Build history of the part. All positions in model axes, mm. Face numbers are marked on the shaded views. A direction names the side the tool comes from. Coordinates: 2 decimals unless noted, no trailing zeros. Loops run counter-clockwise (first coordinate to the right, second up) from the corner with the lowest first, then second, coordinate; pieces in that order, holes last.
Item 1: Cut at A-A (x = 4.5). List the corners of the cut face in (y, z).
Item 2: Cut at B-B (z = 4). List the corners of the cut face in (x, y).
Item 3: 3-axis set-ups, long thin cutter, end or side, ignore diameter. For the marked faces 1, 2 and 3: which of +Z, -Z, +X, -X, +Y, -Y reach the whole face in a straight line?
Item 4: Cut at D-D (x = 0.5). List the corners of the cut face in (y, z).
Item 5: Flat gauge pins, fed straight in: pin 1 (0.6 mm diameter, centred on x = 0.5, y = 17.5, fed in from -Z); pin 2 (1.6 mm diameter, centred on y = 16, z = 16.5, fed in from +X); pin 3 (1.6 mm diameter, centred on x = 4.5, z = 4, fed in from -Y); pin 4 (3.5 mm diameter, centred on y = 15.7, z = 26, fed in from -X). Where does each tip first touch, or does it go through?
Item 6: Mould opens along Y. For the marked faces 4, 5 and 6 say: released by +Y, released by -Y, zero draft, split by the parting line, or undercut.
Item 7: Cut at C-C (z = 20). List the corners of the cut face in (x, y), and give its area (3 significant figures).
Item 8: Drill centre lines: line 1 along Z through (x, y) = (3.6, 15.7); line 2 along Y through (x, z) = (3.25, 25.75); line 3 along Z through (x, y) = (2.75, 16.75). Where is each one in solid material? Low to high.
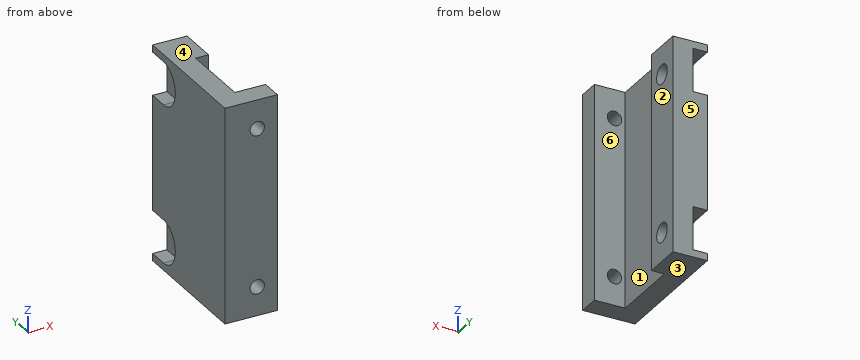
from build123d import *

# Parameters (mm, degrees)
EXTRUDE_1_DEPTH     = 30
CUT_EXTRUDE_1_REACH = 37.994
SKETCH_2_R          = 1
CUT_EXTRUDE_2_REACH = 37.994
SKETCH_3_R          = 1.35
CUT_EXTRUDE_3_DEPTH = 2


with BuildPart() as part:
    # 草图1 → 凸台-拉伸1 (new body)
    with BuildSketch(Plane.XY):
        Polygon((0, 0), (7.3, 0), (7.3, 3), (3, 3), (3, 13), (4.8, 13), (4.8, 18.5), (0, 18.5), align=None)
    extrude(amount=EXTRUDE_1_DEPTH)

    # 草图2 → 切除-拉伸1 (cut, up to next)
    with BuildSketch(Plane.XZ, mode=Mode.PRIVATE) as cut_extrude_1_sk1:
        with Locations((4.5, 26)):
            Circle(SKETCH_2_R)
    cut_extrude_1_tool1 = extrude(cut_extrude_1_sk1.sketch, amount=-CUT_EXTRUDE_1_REACH, mode=Mode.PRIVATE) & part.part
    # 草图2 → 切除-拉伸1 (cut, up to next)
    with BuildSketch(Plane.XZ, mode=Mode.PRIVATE) as cut_extrude_1_sk2:
        with Locations((4.5, 4)):
            Circle(SKETCH_2_R)
    cut_extrude_1_tool2 = extrude(cut_extrude_1_sk2.sketch, amount=-CUT_EXTRUDE_1_REACH, mode=Mode.PRIVATE) & part.part
    add(cut_extrude_1_tool1.solids().sort_by_distance((4.5, 0, 26))[0], mode=Mode.SUBTRACT)
    add(cut_extrude_1_tool2.solids().sort_by_distance((4.5, 0, 4))[0], mode=Mode.SUBTRACT)

    # 草图3 → 切除-拉伸2 (cut, up to next)
    with BuildSketch(Plane.ZY, mode=Mode.PRIVATE) as cut_extrude_2_sk1:
        with Locations(Location((4, 15.7, 0), (0, 0, 270))):
            Circle(SKETCH_3_R)
    cut_extrude_2_tool1 = extrude(cut_extrude_2_sk1.sketch, amount=-CUT_EXTRUDE_2_REACH, mode=Mode.PRIVATE) & part.part
    # 草图3 → 切除-拉伸2 (cut, up to next)
    with BuildSketch(Plane.ZY, mode=Mode.PRIVATE) as cut_extrude_2_sk2:
        with Locations(Location((26, 15.7, 0), (0, 0, 270))):
            Circle(SKETCH_3_R)
    cut_extrude_2_tool2 = extrude(cut_extrude_2_sk2.sketch, amount=-CUT_EXTRUDE_2_REACH, mode=Mode.PRIVATE) & part.part
    add(cut_extrude_2_tool1.solids().sort_by_distance((0, 15.7, 4))[0], mode=Mode.SUBTRACT)
    add(cut_extrude_2_tool2.solids().sort_by_distance((0, 15.7, 26))[0], mode=Mode.SUBTRACT)

    # 草图4 → 切除-拉伸3 (cut)
    with BuildSketch(Plane.ZY):
        with BuildLine():
            Line((1, 15.7), (1, 18.7))
            Line((1, 18.7), (7, 18.7))
            Line((7, 18.7), (7, 15.7))
            ThreePointArc((7, 15.7), (4, 12.7), (1, 15.7))
        make_face()
        with BuildLine():
            Line((23, 15.7), (23, 20.006883846))
            Line((23, 20.006883846), (29, 20.006883846))
            Line((29, 20.006883846), (29, 15.7))
            ThreePointArc((29, 15.7), (26, 12.7), (23, 15.7))
        make_face()
    extrude(amount=-CUT_EXTRUDE_3_DEPTH, mode=Mode.SUBTRACT)


solid = part.part
Filled sheet:
1. outline: (0, 0) - (3, 0) - (3, 3) - (0, 3) - close; (0, 5) - (3, 5) - (3, 25) - (0, 25) - close; (0, 27) - (3, 27) - (3, 30) - (0, 30) - close; (13, 0) - (18.5, 0) - (18.5, 30) - (13, 30) - close; hole circle Ø2.7 at (15.7, 4); hole circle Ø2.7 at (15.7, 26)
2. outline: (0, 0) - (3.5, 0) - (3.5, 3) - (3, 3) - (3, 13) - (4.8, 13) - (4.8, 14.35) - (2, 14.35) - (2, 12.7) - (0, 12.7) - close; (2, 17.05) - (4.8, 17.05) - (4.8, 18.5) - (2, 18.5) - close; (5.5, 0) - (7.3, 0) - (7.3, 3) - (5.5, 3) - close
3. face 1: +Z, -Z, +X
3. face 2: +Z, -Z, +X, +Y
3. face 3: -Z, +X, -X, +Y, -Y
4. outline: (0, 0) - (18.5, 0) - (18.5, 1) - (15.7, 1) arc R3 cw to (15.7, 7) - (18.5, 7) - (18.5, 23) - (15.7, 23) arc R3 cw to (15.7, 29) - (18.5, 29) - (18.5, 30) - (0, 30) - close
5. pin 1: stops at z = 0
5. pin 2: stops at x = 4.8
5. pin 3: stops at y = 13
5. pin 4: stops at x = 2
6. face 4: zero draft
6. face 5: released by +Y
6. face 6: undercut
7. outline: (0, 0) - (7.3, 0) - (7.3, 3) - (3, 3) - (3, 13) - (4.8, 13) - (4.8, 18.5) - (0, 18.5) - close
7. area: 78.3 mm2
8. line 1: z = 0 to 2.65, 5.35 to 24.65, 27.35 to 30
8. line 2: y = 0 to 3, 13 to 14.37, 17.03 to 18.5
8. line 3: z = 0 to 3.15, 4.85 to 25.15, 26.85 to 30
